Here's how the part is built. I have some questions about the finished solid (model axes, mm). A direction names the side the tool comes from. Give positions to 0.01 mm unless a question says otherwise; leave off trailing zeros. Loops run counter-clockwise (first coordinate to the right, second up) from the corner with the lowest first, then second, coordinate; pieces in that order, holes last.
Q1. I'm going to push flat-ended pins straight in: P1, Ø1.3, axis at y = -11.5, z = 3, coming from the +X side; P2, Ø3.5, axis at x = 11.5, z = 3, coming from the -Y side; P3, Ø1.3, axis at x = 13, z = 4, coming from the +Y side; P4, Ø1, axis at y = 8.5, z = 5, coming from the -X side. Where does each tip first touch, or does it pass through?
Q2. Suppose I cut it at B-B (z = 2.55). List the corners of the cut face in (x, y) for me.
Q3. Suppose I cut it at A-A (x = -12). List the corners of the cut face in (y, z) for me.
Q4. For faces 1 (the face through (1, 25.75, 3)), 2 (the face through (5, 32.5, 1)), 3 (the face through (31.25, 0, 4)), 4 (the face through (3, 27.75, 4)), which set-ups out of +Z, -Z, +X, -X, +Y, -Y let a thin tool reach every point of the face, with its end or its side?
Q5. Thinking about a two-plate mould opening in Y: for faces 5 (the face through (2, -25.75, 3)), 6 (the face through (2, -27.75, 4)), 7 (the face through (30, 0, 6)), which applies, pulls with the +Y half, pulls with the -Y half, needs draft (parallel to the pull), parting line crosses it, or undercut?
Q6. I need wall thicknesses on probe 1 along Y at (x, z) = (20.5, 0.8); probe 2 along Y at (x, z) = (6, 3.45); probe 3 along X at (y, z) = (-15, 3.3). Which ranges of each line are inside material? Lowest first, please.
Q7. Suppose I cut it at C-C (y = -2). List the corners of the cut face in (x, z) for me, and give its area (3 significant figures).
```python
from build123d import *

# Parameters (mm, degrees)
F1_DEPTH = 1.5
F2_DEPTH = 6


with BuildPart() as f1:
    # F0 (on Top) → F1 (new body)
    with BuildSketch(Plane.XY):
        Polygon((31.25, -27.75), (-26.318803, -27.75), (-26.318803, -32.5), (35, -32.5), (35, 32.5), (-26.318803, 32.5), (-26.318803, 27.75), (31.25, 27.75), align=None)
        Polygon((29.25, 25.75), (29.25, -25.75), (-26.318803, -25.75), (-26.318803, -27.75), (31.25, -27.75), (31.25, 27.75), (-26.318803, 27.75), (-26.318803, 25.75), align=None)
    extrude(amount=F1_DEPTH)

    # F0 (on Top) → F2 (join)
    with BuildSketch(Plane.XY):
        Polygon((29.25, 25.75), (29.25, -25.75), (-26.318803, -25.75), (-26.318803, -27.75), (31.25, -27.75), (31.25, 27.75), (-26.318803, 27.75), (-26.318803, 25.75), align=None)
    extrude(amount=F2_DEPTH)


solid = f1.part
```
Solutions:
1. P1: stops at x = 31.25
1. P2: stops at y = -32.5
1. P3: stops at y = 27.75
1. P4: stops at x = 29.25
2. outline: (-26.32, -27.75) - (31.25, -27.75) - (31.25, 27.75) - (-26.32, 27.75) - (-26.32, 25.75) - (29.25, 25.75) - (29.25, -25.75) - (-26.32, -25.75) - close
3. outline: (-32.5, 0) - (-25.75, 0) - (-25.75, 6) - (-27.75, 6) - (-27.75, 1.5) - (-32.5, 1.5) - close; (25.75, 0) - (32.5, 0) - (32.5, 1.5) - (27.75, 1.5) - (27.75, 6) - (25.75, 6) - close
4. face 1: +Z, -Z, -X
4. face 2: +Z, -Z, +X, -X, +Y
4. face 3: +Z, +X, +Y, -Y
4. face 4: +Z, +X, -X, +Y
5. face 5: undercut
5. face 6: pulls with the -Y half
5. face 7: needs draft
6. probe 1: y = -32.5 to -25.75, 25.75 to 32.5
6. probe 2: y = -27.75 to -25.75, 25.75 to 27.75
6. probe 3: x = 29.25 to 31.25
7. outline: (29.25, 0) - (35, 0) - (35, 1.5) - (31.25, 1.5) - (31.25, 6) - (29.25, 6) - close
7. area: 17.6 mm2
